Read the model definition and answer for the solid it produces. Units are mm, in the model's axes. A direction names the side the tool comes from. Coordinates: 2 decimals unless noted, no trailing zeros. Loops run counter-clockwise (first coordinate to the right, second up) from the corner with the lowest first, then second, coordinate; pieces in that order, holes last.
from build123d import *

# Parameters (mm, degrees)
F1_DEPTH = 44
F3_DEPTH = 25
F5_D     = 5
F6_SIZE  = 2
F7_SIZE  = 2


with BuildPart() as f1:
    # F0 (on Front) → F1 (new body)
    with BuildSketch(Plane.XZ):
        Polygon((50, 0), (0, 0), (0, -5), (47.668462, -5), (78.309158, -41.51616), (82.13938, -38.302222), align=None)
    extrude(amount=F1_DEPTH)

    # F2 (on face) → F3 (cut)
    with BuildSketch(Plane.XY):
        with BuildLine():
            ThreePointArc((12.776074, -12.236962), (2.776074, -22.236962), (12.776074, -32.236962))
            Line((12.776074, -32.236962), (32.888483, -32.236962))
            ThreePointArc((32.888483, -32.236962), (42.888483, -22.236962), (32.888483, -12.236962))
            Line((32.888483, -12.236962), (12.776074, -12.236962))
        make_face()
    extrude(amount=-F3_DEPTH, mode=Mode.SUBTRACT)

    # F5 (through all)
    with Locations(Plane(origin=(29.341204, 0, 24.620194), x_dir=(0, 1, 0), z_dir=(0.766044, 0, 0.642788))):
        with Locations((-20.821171, -49.455423), (-20.821171, -61.805919)):
            Hole(F5_D / 2)

    # F6
    f6_edges = [f1.edges().sort_by_distance(p)[0] for p in [
        (66.06969, -44, -19.151111),
        (62.98881, -44, -23.25808),
        (78.309158, -22, -41.51616),
        (82.13938, -22, -38.302222),
        (66.06969, 0, -19.151111),
        (62.98881, 0, -23.25808),
    ]]
    chamfer(f6_edges, length=F6_SIZE)

    # F7
    f7_edges = [f1.edges().sort_by_distance(p)[0] for p in [
        (23.694593, 0, 0),
        (23.834231, 0, -5),
        (0, -22, 0),
        (0, -22, -5),
        (23.694593, -44, 0),
        (23.834231, -44, -5),
    ]]
    chamfer(f7_edges, length=F7_SIZE)


solid = f1.part
Q1. A cutting plane is placed at C-C (z = -30). Give the vertices of the cut face in (x, y), then the cut area to 3 significant figures.
Findings below:
outline: (68.65, -42) - (71.26, -44) - (72.56, -44) - (75.17, -42) - (75.17, -2) - (72.56, 0) - (71.26, 0) - (68.65, -2) - close
area: 277 mm2
Q2. Determine the mould class of faces 1 (the face through (78.413, -21.692, -40.106)), 2 (the face through (25, -1, -1)), 3 (the face through (23, -12.237, -2)) for opening direction Y: +Y half, -Y half, draft (parallel to the pull), parting line (faces both ways), or undercut.
Findings below:
face 1: draft
face 2: +Y half
face 3: undercut
Q3. A cutting plane is placed at B-B (y = -8). Give the vertices of the cut face in (x, z), then the cut area to 3 significant figures.
Findings below:
outline: (0, -3) - (2, -5) - (47.67, -5) - (77.02, -39.98) - (79.84, -40.23) - (80.61, -39.59) - (80.85, -36.77) - (50, 0) - (2, 0) - (0, -2) - close
area: 480 mm2
Q4. A cutting plane is placed at A-A (x = 23.5). Give the vertices of the cut face in (y, z), then the cut area to 3 significant figures.
Findings below:
outline: (-44, -3) - (-42, -5) - (-32.24, -5) - (-32.24, 0) - (-42, 0) - (-44, -2) - close; (-12.24, -5) - (-2, -5) - (0, -3) - (0, -2) - (-2, 0) - (-12.24, 0) - close
area: 112 mm2
Q5. Which of the six approach directions +Z, -Z, +X, -X, +Y, -Y give full straight-line access (tool end or side, diameter ignored) to faces 4 (the face through (40.1, -44, -2.6)), 5 (the face through (23, -32.237, -2)), 6 (the face through (25, -8, -5)), 7 (the face through (24, -43, -4))?
Findings below:
face 4: +Z, -Z, +X, -X, -Y
face 5: +Z, -Z
face 6: -Z, -X, +Y, -Y
face 7: -Z, -X, -Y
Q6. Straight lines are drawn through the part: probe 1 along Z at (x, y) = (30, -4); probe 2 along X at (y, z) = (-23, -3); probe 3 along X at (y, z) = (-29, -34.5). For each, find the intervals that lie inside material, in ascending order.
Findings below:
probe 1: z = -5 to 0
probe 2: x = 0 to 2.81, 42.86 to 52.52
probe 3: x = 72.42 to 78.95
Q7. A cutting plane is placed at D-D (x = 35). Give the vertices of the cut face in (y, z), then the cut area to 3 significant figures.
Findings below:
outline: (-44, -3) - (-42, -5) - (-32.01, -5) - (-32.01, 0) - (-42, 0) - (-44, -2) - close; (-12.46, -5) - (-2, -5) - (0, -3) - (0, -2) - (-2, 0) - (-12.46, 0) - close
area: 114 mm2
Q8. Flat-ended cylindrical pins translate along their axes: pin 1 Ø12 at (x, y) = (28, -15) entering from -Z; pin 2 Ø12 at (x, y) = (48, -24.5) entering from -Z; pin 3 Ø5 at (x, z) = (12, -8.5) entering from +Y. Find the tip coordinate at first contact, or state that the pin passes through.
Findings below:
pin 1: stops at z = -5
pin 2: stops at z = -12.55
pin 3: passes through
